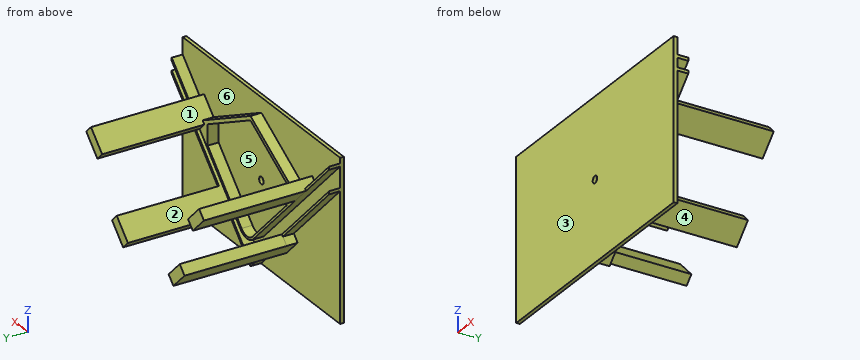
from build123d import *

# Parameters (mm, degrees)
CROQUIS2_W              = 350
CROQUIS2_H              = 220
CROQUIS2_R              = 5
SALIENTE_EXTRUIR1_DEPTH = 20
CORTAR_EXTRUIR1_DEPTH   = 7
CORTAR_EXTRUIR3_DEPTH   = 15
SALIENTE_EXTRUIR3_DEPTH = 140
CORTAR_EXTRUIR4_DEPTH   = 15
SALIENTE_EXTRUIR4_DEPTH = 15


with BuildPart() as part:
    # Croquis2 → Saliente-Extruir1 (new body)
    with BuildSketch(Plane(origin=(0, 0, 0), x_dir=(1, 0, 0), z_dir=(0, 1, 0))):
        Rectangle(CROQUIS2_W, CROQUIS2_H)
        with Locations(Location((0, 0, 0), (0, 0, 270))):
            Circle(CROQUIS2_R, mode=Mode.SUBTRACT)
    extrude(amount=SALIENTE_EXTRUIR1_DEPTH)

    # Croquis3 → Cortar-Extruir1 (cut)
    with BuildSketch(Plane(origin=(0, 20, 0), x_dir=(1, 0, 0), z_dir=(0, 1, 0))):
        Polygon((-7.505553499, 0), (-3.75277675, -6.5), (3.75277675, -6.5), (7.505553499, 0), (3.75277675, 6.5), (-3.75277675, 6.5), align=None)
    extrude(amount=-CORTAR_EXTRUIR1_DEPTH, mode=Mode.SUBTRACT)

    # Croquis8 → Cortar-Extruir3 (cut)
    with BuildSketch(Plane(origin=(0, 20, 0), x_dir=(1, 0, 0), z_dir=(0, 1, 0))):
        with BuildLine():
            Line((21.920310217, 70.351767722), (175, -82.727922061))
            Line((175, -82.727922061), (175, -70))
            Line((175, -70), (0, 105))
            Line((0, 105), (-175, -70))
            Line((-175, -70), (-175, -98.284271247))
            Line((-175, -98.284271247), (-6.363961031, 70.351767722))
            ThreePointArc((-6.363961031, 70.351767722), (7.778174593, 76.209632098), (21.920310217, 70.351767722))
        make_face()
    extrude(amount=-CORTAR_EXTRUIR3_DEPTH, mode=Mode.SUBTRACT)

    # Croquis9 → Saliente-Extruir3 (add)
    with BuildSketch(Plane(origin=(0, 20, 0), x_dir=(1, 0, 0), z_dir=(0, 1, 0))):
        Polygon((-98.994949366, -22.279220614), (-88.388347648, -32.885822331), (-113.13708499, -57.634559673), (-123.743686708, -47.027957955), align=None)
        Polygon((-70.01365227, 34.98634773), (-80.620253988, 45.592949448), (-55.871516646, 70.34168679), (-45.264914928, 59.735085072), align=None)
        Polygon((45.264914928, 59.735085072), (70.01365227, 34.98634773), (80.620253988, 45.592949448), (55.871516646, 70.34168679), align=None)
        Polygon((113.147165922, -20.875087983), (102.540564204, -31.481689701), (127.289301546, -56.230427043), (137.895903264, -45.623825325), align=None)
    extrude(amount=SALIENTE_EXTRUIR3_DEPTH)

    # Croquis10 → Cortar-Extruir4 (cut)
    with BuildSketch(Plane(origin=(0, 20, 0), x_dir=(1, 0, 0), z_dir=(0, 1, 0))):
        Polygon((-175, -65.757359313), (-175, 110), (0, 110), (175, 110), (175, -65.757359313), (72.134972613, 37.107668074), (80.620253988, 45.592949448), (55.871516646, 70.34168679), (47.386235272, 61.856405415), (0, 109.242640687), (-47.386235272, 61.856405415), (-55.871516646, 70.34168679), (-80.620253988, 45.592949448), (-72.134972613, 37.107668074), align=None)
        with BuildLine():
            Line((-96.873629023, -24.400540957), (-88.388347648, -32.885822331))
            Line((-88.388347648, -32.885822331), (-113.13708499, -57.634559673))
            Line((-113.13708499, -57.634559673), (-121.622366364, -49.149278299))
            Line((-121.622366364, -49.149278299), (-175, -102.526911935))
            Line((-175, -102.526911935), (-175, -110))
            Line((-175, -110), (175, -110))
            Line((175, -110), (175, -86.970562748))
            Line((175, -86.970562748), (135.77458292, -47.745145669))
            Line((135.77458292, -47.745145669), (127.289301546, -56.230427043))
            Line((127.289301546, -56.230427043), (102.540564204, -31.481689701))
            Line((102.540564204, -31.481689701), (111.025845579, -22.996408327))
            Line((111.025845579, -22.996408327), (19.798989873, 68.230447378))
            ThreePointArc((19.798989873, 68.230447378), (7.778174593, 73.209632098), (-4.242640687, 68.230447378))
            Line((-4.242640687, 68.230447378), (-96.873629023, -24.400540957))
        make_face()
    extrude(amount=-CORTAR_EXTRUIR4_DEPTH, mode=Mode.SUBTRACT)

    # Croquis11 → Saliente-Extruir4 (add)
    with BuildSketch(Plane(origin=(0, 5, 0), x_dir=(1, 0, 0), z_dir=(0, 1, 0))):
        Polygon((95.070154737, -35.301760182), (95.070154737, -7.040717486), (111.025845579, -22.996408327), (102.540564204, -31.481689701), (106.360634685, -35.301760182), (0, -89.690361331), (-92.048601686, -36.546076369), (-88.388347648, -32.885822331), (-96.873629023, -24.400540957), (-79.786384853, -7.313296787), (-79.786384853, -37.852167867), (0, -83.916858639), align=None)
    extrude(amount=SALIENTE_EXTRUIR4_DEPTH)


solid = part.part
Source: CAD feature listing. Evaluate the final solid. Frame: model axes, mm. Face numbers are marked on the shaded views. A direction names the side the tool comes from. Coordinates: 2 decimals unless noted, no trailing zeros. Order: outer loops, then holes, each group sorted by start corner. A loop starts at its lowest first (then second) coordinate and runs counter-clockwise, first axis right, second up. Notation, with made-up numbers: M -7,-39.75 L 44,-39.75 A32 cw 44,-13.75 Z; hole C 42,29.5 d3. An arc over 180 degrees is marked long. Write each question's results on one line, items separated by ' | '. Start each with the question number.
Item 1: Line query: probe 1 along Z at (x, y) = (0, 2); probe 2 along X at (y, z) = (2.8, 0); probe 3 along Y at (x, z) = (136, 81). Output: solid intervals per line, ascending.
Item 2: Cut plane D-D (x = -104.5). Return loops of the section in (y, z), and give its area (3 significant figures).
Item 3: Cut plane C-C (z = 0). Return loops of the section in (x, y).
Item 4: Cut plane A-A (y = 12.5). Count the separate pieces of the cut face and the enclosed holes in it, and give its area (3 significant figures).
Item 5: Cut plane B-B (y = 85.5). Return loops of the section in (x, z), and give its area (3 significant figures).
Item 6: First-contact query: pin 1 Ø7.5 at (y, z) = (10, 15.5) entering from -X; pin 2 Ø1.5 at (x, z) = (55.5, 8.5) entering from +Y; pin 3 Ø6 at (x, z) = (63.5, -63.5) entering from +Y; pin 4 Ø6 at (x, y) = (-58.5, 71) entering from -Z. Flat tips, straight axial feed; report the tip coordinate or a pass-through.
Item 7: Set-up query: the marked faces 1, 2 and 3. Return all of +Z, -Z, +X, -X, +Y, -Y with unobstructed straight access to the full face (end or side cutting, diameter ignored); none if empty.
Item 8: Draft query along Z for the marked faces 4, 5 and 6. Return one class per face: pulls with the +Z half, pulls with the -Z half, needs draft (parallel to the pull), parting line crosses it, or undercut.
Checked values:
1) probe 1: z = -110 to -5, 5 to 110 | probe 2: x = -175 to -5, 5 to 175 | probe 3: y = 0 to 5
2) outline: M 0,-110 L 5,-110 L 5,-4.74 L 20,-4.74 L 20,-0.5 L 5,-0.5 L 5,27.78 L 160,27.78 L 160,49 L 5,49 L 5,110 L 0,110 Z | area: 4,450 mm2
3) outline: M -175,0 L -5,0 L -5,5 L -72.47,5 L -72.47,20 L -76.72,20 L -76.72,5 L -105,5 L -105,20 L -109.24,20 L -109.24,5 L -175,5 Z; M 5,0 L 175,0 L 175,5 L 109.24,5 L 109.24,20 L 105,20 L 105,5 L 92.27,5 L 92.27,20 L 88.03,20 L 88.03,5 L 5,5 Z
4) separate pieces: 2 | enclosed holes: 1 | area: 6,270 mm2
5) outline: M -123.74,47.03 L -98.99,22.28 L -88.39,32.89 L -113.14,57.63 Z; M -80.62,-45.59 L -55.87,-70.34 L -45.26,-59.74 L -70.01,-34.99 Z; M 45.26,-59.74 L 55.87,-70.34 L 80.62,-45.59 L 70.01,-34.99 Z; M 102.54,31.48 L 113.15,20.88 L 137.9,45.62 L 127.29,56.23 Z | area: 2,100 mm2
6) pin 1: stops at x = -128.49 | pin 2: stops at y = 5 | pin 3: stops at y = 160 | pin 4: stops at z = -70.34
7) face 1: +Z, +Y | face 2: +Y | face 3: +Z, -Z, +X, -X, -Y
8) face 4: pulls with the -Z half | face 5: undercut | face 6: needs draft
